Geometry: final body of the model. Coordinates: model frame, mm. Face numbers are marked on the shaded views. A direction names the side the tool comes from. Give positions to 0.01 mm unless a question says otherwise; leave off trailing zeros. Loops run counter-clockwise (first coordinate to the right, second up) from the corner with the lowest first, then second, coordinate; pieces in that order, holes last.
1. Draft query along Y for the marked faces 3 and 4. Return one class per face: +Y half, -Y half, draft (parallel to the pull), parting line (faces both ways), or undercut.
2. Access query for the marked faces 1 and 2. Directions: +Z, -Z, +X, -X, +Y, -Y. A direction counts if a zero-diameter tool reaches every point of the face in a straight line with its end or side. Return the directions, or none.
3. First-contact query: P1, Ø7.5, axis at x = -127, y = -12.7, coming from the +Z side (3 decimals); P2, Ø1, axis at x = -159, z = 4.5, coming from the +Y side; P3, Ø3, axis at y = 22.5, z = 5, coming from the -X side. Flat tips, straight axial feed; report the tip coordinate or a pass-through.
4. Material intervals for line 1 along Y through (x, z) = (127, 2.1); line 2 along Y through (x, z) = (-127, 5.2) (3 decimals); line 3 along X through (y, z) = (-27, 3.75), sorted ascending.
5. Section A-A, the plane x = 152. Output: boundary loops of the cut face in (y, z) (3 decimals), then the cut area to 3 significant figures.
from build123d import *

# Parameters (mm, degrees)
SKETCH1_W           = 268.605
SKETCH1_H           = 63.5
SKETCH1_R           = 2.286
BOSS_EXTRUDE1_DEPTH = 3.175
SKETCH2_W           = 360.68
SKETCH2_H           = 63.5
SKETCH2_R           = 4.445
BOSS_EXTRUDE2_DEPTH = 3.175
SKETCH3_W           = 12.7
SKETCH3_H           = 25.4
CUT_EXTRUDE1_DEPTH  = 3.175
FILLET1_R           = 2.54
CUT_EXTRUDE2_DEPTH  = 184.223635484
FILLET2_R           = 2.54
SKETCH6_W           = 46.0375
SKETCH6_H           = 12.7
CUT_EXTRUDE3_DEPTH  = 184.141089669


with BuildPart() as part:
    # Sketch1 → Boss-Extrude1 (new body)
    with BuildSketch(Plane.XY):
        Rectangle(SKETCH1_W, SKETCH1_H)
        with Locations((-127, 25.4)):
            Circle(SKETCH1_R, mode=Mode.SUBTRACT)
        with Locations((-127, -12.7)):
            Circle(SKETCH1_R, mode=Mode.SUBTRACT)
        with Locations((-127, -25.4)):
            Circle(SKETCH1_R, mode=Mode.SUBTRACT)
        with Locations(Location((127, 25.4, 0), (0, 0, 180))):
            Circle(SKETCH1_R, mode=Mode.SUBTRACT)
        with Locations(Location((127, -12.7, 0), (0, 0, 180))):
            Circle(SKETCH1_R, mode=Mode.SUBTRACT)
        with Locations(Location((127, -25.4, 0), (0, 0, 180))):
            Circle(SKETCH1_R, mode=Mode.SUBTRACT)
    extrude(amount=BOSS_EXTRUDE1_DEPTH)

    # Sketch2 → Boss-Extrude2 (add)
    with BuildSketch(Plane.XY.offset(3.175)):
        Rectangle(SKETCH2_W, SKETCH2_H)
        with Locations((-127, 25.4)):
            Circle(SKETCH2_R, mode=Mode.SUBTRACT)
        with Locations((-127, -12.7)):
            Circle(SKETCH2_R, mode=Mode.SUBTRACT)
        with Locations((-127, -25.4)):
            Circle(SKETCH2_R, mode=Mode.SUBTRACT)
        with Locations(Location((127, 25.4, 0), (0, 0, 180))):
            Circle(SKETCH2_R, mode=Mode.SUBTRACT)
        with Locations(Location((127, -12.7, 0), (0, 0, 180))):
            Circle(SKETCH2_R, mode=Mode.SUBTRACT)
        with Locations(Location((127, -25.4, 0), (0, 0, 180))):
            Circle(SKETCH2_R, mode=Mode.SUBTRACT)
    extrude(amount=BOSS_EXTRUDE2_DEPTH)

    # Sketch3 → Cut-Extrude1 (cut)
    with BuildSketch(Plane(origin=(0, 0, 0), x_dir=(-1, 0, 0), z_dir=(0, 0, -1))):
        with Locations((-127.9525, 6.35)):
            Rectangle(SKETCH3_W, SKETCH3_H)
        with Locations((127.9525, 6.35)):
            Rectangle(SKETCH3_W, SKETCH3_H)
    extrude(amount=-CUT_EXTRUDE1_DEPTH, mode=Mode.SUBTRACT)

    # Fillet1
    fillet1_edges = [part.edges().sort_by_distance(p)[0] for p in [
        (180.34, 0, 6.35),
        (-180.34, 0, 6.35),
        (-134.3025, 25.4, 0),
        (134.3025, -19.05, 0),
        (134.3025, 25.4, 0),
        (121.6025, 19.05, 1.5875),
        (121.6025, -6.35, 1.5875),
        (-121.6025, 19.05, 1.5875),
        (-121.6025, -6.35, 1.5875),
    ]]
    fillet(fillet1_edges, radius=FILLET1_R)

    # Sketch5 → Cut-Extrude2 (cut, through all)
    with BuildSketch(Plane(origin=(0, 0, 0), x_dir=(-1, 0, 0), z_dir=(0, 0, -1))):
        with BuildLine():
            Line((-27.124304603, 1.369033584), (-38.1, -31.75))
            Line((-38.1, -31.75), (38.1, -31.75))
            Line((38.1, -31.75), (27.124304603, 1.369033584))
            ThreePointArc((27.124304603, 1.369033584), (0, 20.955), (-27.124304603, 1.369033584))
        make_face()
    extrude(amount=-CUT_EXTRUDE2_DEPTH, mode=Mode.SUBTRACT)

    # Fillet2
    fillet2_edges = [part.edges().sort_by_distance(p)[0] for p in [
        (0, 20.955, 6.35),
        (-32.612152302, -15.190483208, 6.35),
        (-38.1, -31.75, 3.175),
        (32.612152302, -15.190483208, 6.35),
        (38.1, -31.75, 3.175),
        (0, 20.955, 0),
        (32.612152302, -15.190483208, 0),
        (-32.612152302, -15.190483208, 0),
    ]]
    fillet(fillet2_edges, radius=FILLET2_R)

    # Sketch6 → Cut-Extrude3 (cut, through all)
    with BuildSketch(Plane(origin=(0, 0, 3.175), x_dir=(-1, 0, 0), z_dir=(0, 0, -1))):
        with Locations((-157.32125, 25.4)):
            Rectangle(SKETCH6_W, SKETCH6_H)
        with Locations((157.32125, 25.4)):
            Rectangle(SKETCH6_W, SKETCH6_H)
    extrude(amount=-CUT_EXTRUDE3_DEPTH, mode=Mode.SUBTRACT)


solid = part.part
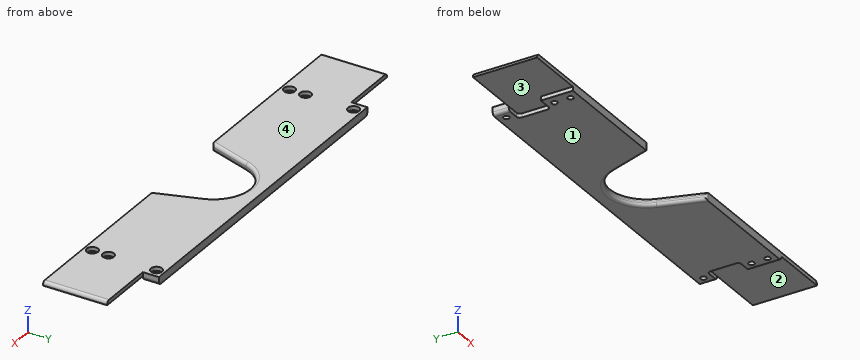
Answers below:
1. face 3: undercut
1. face 4: draft
2. face 1: -Z, +X, -X, +Y, -Y
2. face 2: -Z, +X
3. P1: stops at z = 3.175
3. P2: stops at y = 19.05
3. P3: stops at x = -134.3
4. line 1: y = -31.75 to -27.69, -23.11 to -14.99, -10.41 to -6.35, 19.05 to 23.11, 27.69 to 31.75
4. line 2: y = -31.75 to -29.845, -20.955 to -17.145, -8.255 to 20.955, 29.845 to 31.75
4. line 3: x = -180.34 to -131.15, -122.85 to -36.53, 36.53 to 122.85, 131.15 to 180.34
5. outline: (-31.75, 3.175) - (19.05, 3.175) - (19.05, 6.35) - (-31.75, 6.35) - close
5. area: 161 mm2
